Check sheet for the modelled part. Datum: model origin and axes. Units: mm. Give positions to 0.01 mm unless a question says otherwise; leave off trailing zeros. Write each loop counter-clockwise with the first axis right and the second up, starting at its lowest first coordinate (ties: lowest second). Pieces come first, ordered by that corner, then holes. Notation, with made-up numbers: (73.5, 34) -> (87.5, 34) arc R25 cw to (87.5, 53) -> close; hole circle Ø10 at (27, 21.25). An arc over 180 degrees is marked (long way). Write each question's results on one line, items separated by ' | '. Start each with the question number.
```python
from build123d import *


with BuildPart() as part:
    # Sketch2 → Revolve2 (revolve)
    with BuildSketch(Plane.XY, mode=Mode.PRIVATE) as revolve2_sk:
        with BuildLine():
            Line((0, 0), (0, 10.034926072))
            Line((0, 10.034926072), (-15.174290575, 10.034926072))
            ThreePointArc((-15.174290575, 10.034926072), (-17.033998604, 9.069882685), (-17.78, 7.112))
            Line((-17.78, 7.112), (-17.78, 4.572))
            ThreePointArc((-17.78, 4.572), (-17.640170395, 4.132059095), (-17.272, 3.85357951))
            Line((-17.272, 3.85357951), (-17.272, 3.76642049))
            ThreePointArc((-17.272, 3.76642049), (-17.640170395, 3.487940905), (-17.78, 3.048))
            Line((-17.78, 3.048), (-17.78, 0.762))
            ThreePointArc((-17.78, 0.762), (-17.556815367, 0.223184633), (-17.018, 0))
            Line((-17.018, 0), (0, 0))
        make_face()
    revolve(revolve2_sk.sketch.rotate(Axis((0, 0, 0), (0, 1, 0)), 270), axis=Axis((0, 0, 0), (0, 1, 0)))


solid = part.part
```
Item 1: Section check A-A on y = 5.25. Record the boundary of the cut face in (x, z).
Item 2: Thickness scan on probe 1 along Z at (x, y) = (-0.5, 8.75); probe 2 along Z at (x, y) = (11, 7.25); probe 3 along X at (y, z) = (7.5, 6). Record the ranges inside material, lowest first. Write a range as from..to.
Item 3: Depth check by flat-ended pin: pin 1 Ø6 at (x, y) = (-4, 8.5) entering from -Z; pin 2 Ø4 at (x, y) = (12.5, 8.5) entering from -Z; pin 3 Ø2 at (x, y) = (13.5, 3.5) entering from +Z. Enter the tip coordinate at first touch or a pass-through.
Item 4: Section check B-B on y = 8.5. Record the boundary of the cut face in (x, z).
Check sheet entries:
1) outline: circle Ø35.56 at (0, 0)
2) probe 1: z = -17.27..17.27 | probe 2: z = -13.96..13.96 | probe 3: x = -16.71..16.71
3) pin 1: stops at z = -17.73 | pin 2: stops at z = -14.15 | pin 3: stops at z = 12.58
4) outline: circle Ø34.86 at (0, 0)
